Part model, mm, in its own coordinate system. Face numbers are marked on the shaded views. Round coordinates to 2 decimals unless told otherwise and drop trailing zeros. Write each loop counter-clockwise with the first axis right and the second up, starting at its lowest first coordinate (ties: lowest second). Pieces come first, ordered by that corner, then holes.
1) Flat gauge pins, fed straight in: pin 1 (1.3 mm diameter, centred on x = 1.118, y = -7.62, fed in from -Z); pin 2 (0.6 mm diameter, centred on x = -3.962, y = -7.62, fed in from +Z); pin 3 (0.9 mm diameter, centred on x = -6, y = 2.5, fed in from +Z); pin 4 (0.5 mm diameter, centred on x = -3.5, z = 1, fed in from +Y). Where does each tip first touch, or does it go through?
2) Saw through at B-B on x = -3. Write the cut outline in (y, z) (3 decimals), and give its area (3 significant figures).
3) Drill centre lines: L1, parallel to Y at x = 1.25, z = 0.2; L2, parallel to Y at x = 0.75, z = 0.05; L3, parallel to Z at x = 0, y = -4.75. Where is each one in solid material? Low to high.
4) Pull direction Y, two halves, no side cores. Call the marked faces 1, 2 and 3: +Y half, -Y half, draft (parallel to the pull), parting line (faces both ways), or undercut.
5) Saw through at D-D on y = 6.5. Write the cut outline in (x, z), and give its area (3 significant figures).
6) Saw through at A-A on y = 0. Write the cut outline in (x, z) (3 decimals).
7) Saw through at C-C on z = -0.5. Count the separate pieces of the cut face and the enclosed holes in it, and give its area (3 significant figures).
```python
from build123d import *

# Parameters (mm, degrees)
F0_W     = 17.018
F0_H     = 17.78
F1_DEPTH = 0.26
F2_DEPTH = 1.35
F3_R     = 0.508
F3_R_2   = 0.509027
F3_R_3   = 0.487745
F3_R_4   = 1.651
F4_DEPTH = 1.61
F5_W     = 1.6
F5_H     = 0.8
F5_W_2   = 0.8
F5_H_2   = 1.6
F6_DEPTH = 0.5
F7_W     = 4
F7_H     = 4
F8_DEPTH = 1.075


with BuildPart() as f1:
    # F0 (on Top) → F1 (new body)
    with BuildSketch(Plane.XY):
        Rectangle(F0_W, F0_H)
    extrude(amount=F1_DEPTH)

    # F0 (on Top) → F2 (join)
    with BuildSketch(Plane.XY):
        Rectangle(F0_W, F0_H)
    extrude(amount=-F2_DEPTH)

    # F3 (on face) → F4 (cut, through all)
    with BuildSketch(Plane.XY.offset(0.26)):
        with Locations((-6.502, 7.62)):
            Circle(F3_R)
        with Locations((-3.962, 7.62)):
            Circle(F3_R)
        with Locations((-1.422, 7.62)):
            Circle(F3_R)
        with Locations((1.118, 7.62)):
            Circle(F3_R)
        with Locations((1.118, 2.54)):
            Circle(F3_R)
        with Locations((1.118, 0)):
            Circle(F3_R)
        with Locations((1.123042, -2.550522)):
            Circle(F3_R_2)
        with Locations((1.118, -7.62)):
            Circle(F3_R)
        with Locations((-1.401745, -7.62)):
            Circle(F3_R_3)
        with Locations((-3.962, -7.62)):
            Circle(F3_R)
        with Locations((-6.502, -7.62)):
            Circle(F3_R)
        with Locations((5.715, -6.096)):
            Circle(F3_R_4)
        with Locations((5.715, 6.096)):
            Circle(F3_R_4)
    extrude(amount=-F4_DEPTH, mode=Mode.SUBTRACT)

    # F5 (on face) → F6 (join)
    with BuildSketch(Plane.XY.offset(0.26)):
        with Locations((-6.579, 5.334)):
            Rectangle(F5_W, F5_H)
        with Locations((-6.579, 4.064)):
            Rectangle(F5_W, F5_H)
        with Locations((-6.579, 2.794)):
            Rectangle(F5_W, F5_H)
        with Locations((-1.016, -0.152)):
            Rectangle(F5_W_2, F5_H_2)
        with Locations((-3.759, -4.064)):
            Rectangle(F5_W_2, F5_H_2)
    extrude(amount=F6_DEPTH)

    # F7 (on face) → F8 (join)
    with BuildSketch(Plane.XY.offset(0.26)):
        with Locations((-3.962, 0)):
            Rectangle(F7_W, F7_H)
    extrude(amount=F8_DEPTH)


solid = f1.part
```
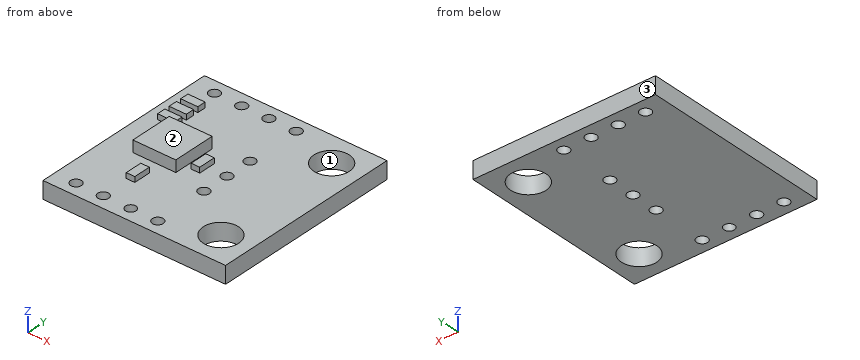
Completed:
1. pin 1: stops at z = -1.35
1. pin 2: passes through
1. pin 3: stops at z = 0.76
1. pin 4: stops at y = 2
2. outline: (-8.89, -1.35) - (8.89, -1.35) - (8.89, 0.26) - (2, 0.26) - (2, 1.335) - (-2, 1.335) - (-2, 0.26) - (-8.89, 0.26) - close
2. area: 32.9 mm2
3. L1: y = -8.89 to -8.11, -7.13 to -3.04, -2.06 to -0.49, 0.49 to 2.05, 3.03 to 7.13, 8.11 to 8.89
3. L2: y = -8.89 to -7.97, -7.27 to -2.9, -2.2 to -0.35, 0.35 to 2.19, 2.89 to 7.27, 7.97 to 8.89
3. L3: z = -1.35 to 0.26
4. face 1: undercut
4. face 2: draft
4. face 3: +Y half
5. outline: (-8.51, -1.35) - (4.11, -1.35) - (4.11, 0.26) - (-8.51, 0.26) - close; (7.32, -1.35) - (8.51, -1.35) - (8.51, 0.26) - (7.32, 0.26) - close
5. area: 22.2 mm2
6. outline: (-8.509, -1.35) - (0.61, -1.35) - (0.61, 0.26) - (-0.616, 0.26) - (-0.616, 0.76) - (-1.416, 0.76) - (-1.416, 0.26) - (-1.962, 0.26) - (-1.962, 1.335) - (-5.962, 1.335) - (-5.962, 0.26) - (-8.509, 0.26) - close; (1.626, -1.35) - (8.509, -1.35) - (8.509, 0.26) - (1.626, 0.26) - close
7. separate pieces: 1
7. enclosed holes: 13
7. area: 277 mm2
